For this review, take the finished solid that the model builds, in its own axes (mm). A direction names the side the tool comes from. Round coordinates to 2 decimals unless told otherwise and drop trailing zeros. Order: outer loops, then holes, each group sorted by start corner. A loop starts at its lowest first (then second) coordinate and runs counter-clockwise, first axis right, second up. Notation, with made-up numbers: (73.25, 3) - (105.25, 3) arc R20 cw to (105.25, 12) - close; hole circle Ø8 at (2.25, -37). An arc over 180 degrees is marked (long way). Write each question's results on one line, items separated by ' | '. Start each with the question number.
(1) Take a section at C-C, the plane z = 27.25. Give the boundary of the cut face in (x, y), plus the area to 3 significant figures.
(2) For faces 1 (the cylindrical face through (15.317, -0.986, 22.473)), 2 (the flat face through (5, -1, 29.665)), 3 (the flat face through (-6, -2, 16)), list the 3-axis set-ups (+Z, -Z, +X, -X, +Y, -Y) from which the entire face can be reached by the end or side of a thin tool; tool diameter is ignored.
(3) For L1, parallel to Z at x = 9, y = -4.15; L2, parallel to X at y = -3.9, z = 27.75; L3, parallel to X at y = -4.2, z = 14.5, list the stretches that pass through material, from the lowest coordinate up. Write a range as from..to.
(4) Draft analysis for pull direction Z (two halves, no side actions). For faces 4 (the flat face through (13, -1, 4.665)), 5 (the flat face through (-9.7, -5, 25.5)), 6 (the flat face through (18.686, -4, 11)), 7 (the flat face through (13, -3, 30.165)), state which applies: pulls with the +Z half, pulls with the -Z half, needs draft (parallel to the pull), parting line crosses it, or undercut.
(5) Insertion check: pin 1 Ø2 at (x, y) = (13, -0.5) entering from -Z; pin 2 Ø9 at (x, z) = (20.69, 23.66) entering from -Y; pin 3 Ø1.6 at (x, y) = (5.5, -1) entering from +Z; pin 4 Ø1 at (x, y) = (-2, -3.5) entering from -Z. Each pin has a flat end and moves straight along its axis. Give the tip position at first contact, or say it passes through.
(6) Take a section at B-B, the plane x = 25. Give the boundary of the cut face in (y, z).
(7) Take a section at D-D, the plane x = 47. Give the boundary of the cut face in (y, z), plus the area to 3 significant figures.
(8) Take a section at A-A, the plane x = -5. Give the boundary of the cut face in (y, z), plus the area to 3 significant figures.
```python
from build123d import *

# Parameters (mm, degrees)
SKETCH1_R               = 5.5
BOSS_EXTRUDE1_DEPTH     = 2
BOSS_EXTRUDE1_2_DEPTH   = 2
BOSS_EXTRUDE1_3_DEPTH   = 2
BOSS_EXTRUDE1_4_DEPTH   = 2
BOSS_EXTRUDE1_5_DEPTH   = 2
BOSS_EXTRUDE1_6_DEPTH   = 2
BOSS_EXTRUDE2_START     = -5
BOSS_EXTRUDE2_OUTLINE_R = 1.7
BOSS_EXTRUDE2_DEPTH     = 5
CUT_EXTRUDE1_DEPTH      = 1


# Read off the part's stored shape, not the designer's step: Boss-Extrude2
with BuildPart() as part:
    # Sketch1 → Boss-Extrude1 (new body)
    with BuildSketch(Plane(origin=(0, 0, 0), x_dir=(1, 0, 0), z_dir=(0, 1, 0))):
        Polygon((2.686395113, -16.66487452), (2.68639507, -4.66487452), (-9.31360493, -4.664874562), (-9.313604887, -16.664874562), align=None)
        with Locations(Location((-3.313604908, -10.664874541, 0), (0, 0, 270))):
            Circle(SKETCH1_R, mode=Mode.SUBTRACT)
    extrude(amount=-BOSS_EXTRUDE1_DEPTH)



with BuildPart() as body_2:
    # Sketch1 → Boss-Extrude1 2 (new body)
    with BuildSketch(Plane(origin=(0, 0, 0), x_dir=(1, 0, 0), z_dir=(0, 1, 0))):
        Polygon((18.686395113, -16.664873819), (18.68639507, -4.664873819), (6.68639507, -4.664873862), (6.686395113, -16.664873862), align=None)
        with Locations(Location((12.686395092, -10.66487384, 0), (0, 0, 270))):
            Circle(SKETCH1_R, mode=Mode.SUBTRACT)
    extrude(amount=-BOSS_EXTRUDE1_2_DEPTH)


with BuildPart() as body_3:
    # Sketch1 → Boss-Extrude1 3 (new body)
    with BuildSketch(Plane(origin=(0, 0, 0), x_dir=(1, 0, 0), z_dir=(0, 1, 0))):
        Polygon((34.686395113, -16.664873762), (34.68639507, -4.664873762), (22.68639507, -4.664873805), (22.686395113, -16.664873805), align=None)
        with Locations(Location((28.686395092, -10.664873784, 0), (0, 0, 270))):
            Circle(SKETCH1_R, mode=Mode.SUBTRACT)
    extrude(amount=-BOSS_EXTRUDE1_3_DEPTH)


with BuildPart() as body_4:
    # Sketch1 → Boss-Extrude1 4 (new body)
    with BuildSketch(Plane(origin=(0, 0, 0), x_dir=(1, 0, 0), z_dir=(0, 1, 0))):
        Polygon((14.68639512, -17.664873833), (14.686395163, -29.664873833), (26.686395163, -29.664873791), (26.68639512, -17.664873791), align=None)
        with Locations(Location((20.686395141, -23.664873812, 0), (0, 0, 270))):
            Circle(SKETCH1_R, mode=Mode.SUBTRACT)
    extrude(amount=-BOSS_EXTRUDE1_4_DEPTH)


with BuildPart() as body_5:
    # Sketch1 → Boss-Extrude1 5 (new body)
    with BuildSketch(Plane(origin=(0, 0, 0), x_dir=(1, 0, 0), z_dir=(0, 1, 0))):
        Polygon((-1.31360488, -17.664873456), (-1.313604837, -29.664873456), (10.686395163, -29.664873413), (10.68639512, -17.664873413), align=None)
        with Locations(Location((4.686395141, -23.664873434, 0), (0, 0, 270))):
            Circle(SKETCH1_R, mode=Mode.SUBTRACT)
    extrude(amount=-BOSS_EXTRUDE1_5_DEPTH)


with BuildPart() as body_6:
    # Sketch1 → Boss-Extrude1 6 (new body)
    with BuildSketch(Plane(origin=(0, 0, 0), x_dir=(1, 0, 0), z_dir=(0, 1, 0))):
        Polygon((30.68639512, -17.664873979), (30.686395163, -29.664873979), (42.686395163, -29.664873936), (42.68639512, -17.664873936), align=None)
        with Locations(Location((36.686395141, -23.664873958, 0), (0, 0, 270))):
            Circle(SKETCH1_R, mode=Mode.SUBTRACT)
    extrude(amount=-BOSS_EXTRUDE1_6_DEPTH)


with BuildPart() as part_1:
    add(part.part)

    add(body_2.part)  # Boss-Extrude2 merges body 2

    add(body_3.part)  # Boss-Extrude2 merges body 3

    add(body_4.part)  # Boss-Extrude2 merges body 4

    add(body_5.part)  # Boss-Extrude2 merges body 5

    add(body_6.part)  # Boss-Extrude2 merges body 6
    # Boss-Extrude2 outline → Boss-Extrude2 (add)
    with BuildSketch(Plane(origin=(0, 0, 0), x_dir=(1, 0, 0), z_dir=(0, 1, 0)).offset(BOSS_EXTRUDE2_START)):
        Polygon((42.686395163, -29.664873936), (39.186395163, -29.664873949), (39.186395164, -30.164873949), (52.686395098, -30.16487344), (52.686395098, -4.164874546), (31.186395069, -4.164873775), (31.18639507, -4.664873775), (34.68639507, -4.664873762), (34.686395113, -16.664873762), (22.686395113, -16.664873805), (22.68639507, -4.664873805), (26.186395069, -4.664873793), (26.186395069, -4.164873793), (15.186395069, -4.164873832), (15.18639507, -4.664873832), (18.68639507, -4.664873819), (18.686395113, -16.664873819), (6.686395113, -16.664873862), (6.68639507, -4.664873862), (10.186395069, -4.664873849), (10.186395069, -4.164873849), (-0.813604931, -4.164873888), (-0.81360493, -4.664874532), (2.68639507, -4.66487452), (2.686395113, -16.66487452), (-9.313604887, -16.664874562), (-9.31360493, -4.664874562), (-5.813604931, -4.66487455), (-5.813604931, -4.16487455), (-19.313604998, -4.164874546), (-19.313604998, -30.16487344), (2.186395164, -30.164873443), (2.186395163, -29.664873443), (-1.313604837, -29.664873456), (-1.31360488, -17.664873456), (10.68639512, -17.664873413), (10.686395163, -29.664873413), (7.186395163, -29.664873425), (7.186395164, -30.164873425), (18.186395164, -30.164873821), (18.186395163, -29.664873821), (14.686395163, -29.664873833), (14.68639512, -17.664873833), (26.68639512, -17.664873791), (26.686395163, -29.664873791), (23.186395163, -29.664873803), (23.186395164, -30.164873803), (34.186395164, -30.164873764), (34.186395163, -29.664873966), (30.686395163, -29.664873979), (30.68639512, -17.664873979), (42.68639512, -17.664873936), align=None)
        with Locations((-14.313604998, -17.164873993)):
            Circle(BOSS_EXTRUDE2_OUTLINE_R, mode=Mode.SUBTRACT)
        with Locations((47.686395098, -17.164873993)):
            Circle(BOSS_EXTRUDE2_OUTLINE_R, mode=Mode.SUBTRACT)
    extrude(amount=BOSS_EXTRUDE2_DEPTH)

    # Sketch2 → Cut-Extrude1 (cut)
    # profile 1 of 2: a face of its own
    with BuildSketch(Plane(origin=(0, -5, 0), x_dir=(-1, 0, 0), z_dir=(0, -1, 0))):
        Polygon((6.699801581, -23.2390136), (8.246596453, -23.2390136), (8.246596453, -23.564654626), (6.984737478, -23.564654626), (6.984737478, -24.541577703), (8.246596453, -24.541577703), (8.246596453, -24.867218728), (6.984737478, -24.867218728), (6.984737478, -26.4140136), (6.699801581, -26.4140136), align=None)
    # profile 2 of 2: a face of its own
    with BuildSketch(Plane(origin=(0, -5, 0), x_dir=(-1, 0, 0), z_dir=(0, -1, 0))):
        with BuildLine():
            Line((9.996916965, -23.157603344), (10.216979065, -23.329964121))
            Line((10.216979065, -23.329964121), (9.378071813, -24.612811677))
            add(Edge.make_bspline(
                [(9.378071813, -24.612811677), (9.43392485, -24.603909103), (9.542872514, -24.586543627), (9.65315015, -24.583678919), (9.706892927, -24.582282831)],
                knots=[0, 0, 0, 0, 1.025318673, 2, 2, 2, 2], degree=3))
            add(Edge.make_bspline(
                [(9.706892927, -24.582282831), (9.739163887, -24.583137599), (9.802478203, -24.584814619), (9.895509725, -24.598067595), (9.984924431, -24.618695779), (10.070522851, -24.64888638), (10.152413619, -24.68743998), (10.231065003, -24.733649384), (10.30499899, -24.789897237), (10.375167554, -24.852730491), (10.438873565, -24.922323744), (10.49527613, -24.996166388), (10.542653291, -25.074181472), (10.581092491, -25.156329486), (10.610941917, -25.2424838), (10.632702138, -25.332534184), (10.645565054, -25.426542733), (10.647311749, -25.490476506), (10.648199017, -25.522952903)],
                knots=[0, 0, 0, 0, 1.044136307, 2.048553127, 3.035567123, 4.010001674, 4.980053131, 5.96154148, 6.956538004, 7.981742224, 9.006487041, 10.005615874, 10.984750588, 11.954802044, 12.935714515, 13.930994945, 14.949008866, 16, 16, 16, 16], degree=3))
            add(Edge.make_bspline(
                [(10.648199017, -25.522952903), (10.646908057, -25.567384491), (10.644367755, -25.654815343), (10.619055025, -25.782157069), (10.579721633, -25.903471565), (10.523499161, -26.016821942), (10.453665142, -26.122052845), (10.368504755, -26.215293946), (10.271038162, -26.298451765), (10.160832281, -26.36799027), (10.042229735, -26.42478018), (9.917631851, -26.465570078), (9.788248654, -26.49068294), (9.700433045, -26.493831272), (9.656011517, -26.495423856)],
                knots=[0, 0, 0, 0, 1.031375318, 2.029502543, 3.004789286, 3.987476834, 4.960371455, 5.9300674, 6.912260825, 7.929083631, 8.949397511, 9.960523116, 10.96833055, 12, 12, 12, 12], degree=3))
            add(Edge.make_bspline(
                [(9.656011517, -26.495423856), (9.613288081, -26.494037555), (9.528660436, -26.491291536), (9.404170686, -26.466829578), (9.284552092, -26.427180992), (9.170642725, -26.372558039), (9.065123312, -26.303562674), (8.970720913, -26.220502607), (8.887906232, -26.125153306), (8.818986397, -26.017529563), (8.764323119, -25.901877958), (8.723329401, -25.781284966), (8.699384238, -25.656189983), (8.69603819, -25.571389235), (8.694352863, -25.528677062)],
                knots=[0, 0, 0, 0, 1.012016664, 2.004627821, 2.994792927, 3.992885782, 4.990978636, 5.973936114, 6.964471063, 7.975201453, 8.993600317, 9.990122807, 10.98767138, 12, 12, 12, 12], degree=3))
            add(Edge.make_bspline(
                [(8.694352863, -25.528677062), (8.695424602, -25.495979475), (8.697612889, -25.429217252), (8.712892251, -25.328103455), (8.737443886, -25.224642831), (8.764939609, -25.136872955), (8.793991413, -25.064971432), (8.818169074, -25.007001837), (8.848262627, -24.947347149), (8.880351337, -24.883961779), (8.91732364, -24.818479279), (8.957524265, -24.749805236), (9.002064662, -24.679031831), (9.033288667, -24.631003882), (9.049250699, -24.606451501)],
                knots=[0, 0, 0, 0, 1.173818275, 2.396712641, 3.66331629, 4.989737886, 5.693666774, 6.447286557, 7.243889047, 8.091586357, 8.998013824, 9.943181721, 10.948533338, 12, 12, 12, 12], degree=3))
            Line((9.049250699, -24.606451501), (9.996916965, -23.157603344))
        make_face()
        with BuildLine():
            add(Edge.make_bspline(
                [(9.64710727, -24.907923856), (9.622921579, -24.908639019), (9.575469451, -24.910042162), (9.505937895, -24.917966716), (9.440309411, -24.932982832), (9.377830069, -24.952402516), (9.31916676, -24.978858553), (9.263592246, -25.010560401), (9.211746157, -25.048541998), (9.16388158, -25.091418934), (9.120507249, -25.138406483), (9.083148796, -25.188723076), (9.050925237, -25.241169384), (9.024725214, -25.296180139), (9.004323526, -25.353735218), (8.989565892, -25.413569669), (8.981352848, -25.476084793), (8.97998648, -25.518477849), (8.97928876, -25.540125379)],
                knots=[0, 0, 0, 0, 1.128956033, 2.215002439, 3.259141796, 4.2666399, 5.263148119, 6.255916712, 7.247353359, 8.256307737, 9.250603402, 10.226115518, 11.176314381, 12.118911324, 13.063945463, 14.021379252, 14.989639887, 16, 16, 16, 16], degree=3))
            add(Edge.make_bspline(
                [(8.97928876, -25.540125379), (8.97985696, -25.561579289), (8.980971114, -25.603647213), (8.991087861, -25.665640612), (9.006541115, -25.725298779), (9.029528474, -25.782314158), (9.056948579, -25.837555818), (9.093148409, -25.889022827), (9.133259351, -25.939841033), (9.181205419, -25.986106654), (9.232661612, -26.029156591), (9.28763556, -26.066785107), (9.344930667, -26.098976136), (9.405320457, -26.124204774), (9.467948134, -26.144909663), (9.533335493, -26.159479719), (9.601528012, -26.167717054), (9.647721485, -26.169085201), (9.67127594, -26.169782831)],
                knots=[0, 0, 0, 0, 0.989467248, 1.94019797, 2.891935182, 3.827694429, 4.772920941, 5.730924762, 6.725747692, 7.756678648, 8.79901574, 9.819492441, 10.826891316, 11.826466727, 12.835195252, 13.867842842, 14.912794438, 16, 16, 16, 16], degree=3))
            add(Edge.make_bspline(
                [(9.67127594, -26.169782831), (9.694830356, -26.169085146), (9.741023753, -26.167716892), (9.809216821, -26.159480335), (9.874602152, -26.144907404), (9.9372372, -26.124212963), (9.997599783, -26.09894576), (10.054844781, -26.066985375), (10.109298837, -26.028925183), (10.16078881, -25.986180223), (10.208535311, -25.939577707), (10.249608271, -25.889476459), (10.28469949, -25.837139854), (10.313214788, -25.782531768), (10.335948959, -25.725264304), (10.351480576, -25.665649848), (10.361576431, -25.603644795), (10.362693456, -25.561578473), (10.363263119, -25.540125379)],
                knots=[0, 0, 0, 0, 1.087397944, 2.132534446, 3.165364764, 4.174271784, 5.174024072, 6.181601208, 7.194203697, 8.236725232, 9.267838612, 10.269026844, 11.221737037, 12.171628256, 13.107553087, 14.05945871, 15.010357665, 16, 16, 16, 16], degree=3))
            add(Edge.make_bspline(
                [(10.363263119, -25.540125379), (10.362763924, -25.518449609), (10.361784167, -25.475907121), (10.350702565, -25.413597625), (10.335333378, -25.35343124), (10.31212604, -25.29578579), (10.28197527, -25.240889945), (10.245252874, -25.18846183), (10.202761835, -25.138117296), (10.153715725, -25.091298499), (10.100325283, -25.048806355), (10.043918117, -25.010417813), (9.98414317, -24.979153645), (9.922078942, -24.95231253), (9.856977887, -24.933290658), (9.789551091, -24.917919833), (9.719159645, -24.910108409), (9.671290808, -24.908657076), (9.64710727, -24.907923856)],
                knots=[0, 0, 0, 0, 0.978753431, 1.920974676, 2.853199117, 3.782215702, 4.721507756, 5.67862441, 6.671401678, 7.694929396, 8.738190014, 9.75360867, 10.774035531, 11.783329636, 12.805060902, 13.835252836, 14.906360638, 16, 16, 16, 16], degree=3))
        make_face(mode=Mode.SUBTRACT)
    extrude(amount=-CUT_EXTRUDE1_DEPTH, mode=Mode.SUBTRACT)


solid = part_1.part
```
Results below:
1) outline: (-19.31, -5) - (-1.31, -5) - (-1.31, -2) - (0.52, -2) - (0.52, 0) - (-19.31, 0) - close; (8.86, -2) - (10.69, -2) - (10.69, -5) - (14.69, -5) - (14.69, -2) - (16.52, -2) - (16.52, 0) - (8.86, 0) - close; (24.86, -2) - (26.69, -2) - (26.69, -5) - (30.69, -5) - (30.69, -2) - (32.52, -2) - (32.52, 0) - (24.86, 0) - close; (40.86, -2) - (42.69, -2) - (42.69, -5) - (52.69, -5) - (52.69, 0) - (40.86, 0) - close | area: 202 mm^2
2) face 1: +Y, -Y | face 2: +Z, +Y, -Y | face 3: -Y
3) L1: z = 4.16..4.66, 16.66..17.66, 29.66..30.16 | L2: x = -19.31..-1.31, 10.69..14.69, 26.69..30.69, 42.69..52.69 | L3: x = -19.31..-9.31, 2.69..6.69, 18.69..22.69, 34.69..52.69
4) face 4: pulls with the -Z half | face 5: needs draft | face 6: undercut | face 7: pulls with the +Z half
5) pin 1: stops at z = 4.66 | pin 2: passes through | pin 3: stops at z = 29.66 | pin 4: stops at z = 16.66
6) outline: (-5, 4.16) - (0, 4.16) - (0, 6.58) - (-2, 6.58) - (-2, 4.66) - (-5, 4.66) - close; (-5, 16.66) - (-2, 16.66) - (-2, 14.75) - (0, 14.75) - (0, 20.25) - (-2, 20.25) - (-2, 17.66) - (-5, 17.66) - close; (-5, 29.66) - (-2, 29.66) - (-2, 27.08) - (0, 27.08) - (0, 30.16) - (-5, 30.16) - close
7) outline: (-5, 4.16) - (0, 4.16) - (0, 15.61) - (-5, 15.61) - close; (-5, 18.72) - (0, 18.72) - (0, 30.16) - (-5, 30.16) - close | area: 114 mm^2
8) outline: (-5, 16.66) - (-2, 16.66) - (-2, 15.9) - (0, 15.9) - (0, 30.16) - (-5, 30.16) - close; (-2, 4.66) - (0, 4.66) - (0, 5.43) - (-2, 5.43) - close | area: 70.6 mm^2
